Here's how the part is built. I have some questions about the finished solid (model axes, mm). Give positions to 0.01 mm unless a question says otherwise; leave off trailing zeros. Loops run counter-clockwise (first coordinate to the right, second up) from the corner with the lowest first, then second, coordinate; pieces in that order, holes last. Notation, with made-up numbers: (-24.75, 25) - (34.25, 25) arc R22 cw to (34.25, 40) - close; hole circle Ø8 at (77.5, 5.25). An arc over 180 degrees is marked (long way). Put each result on its own line as item: value. Start each with the question number.
from build123d import *

# Parameters (mm, degrees)
CROQUIS1_W              = 33.201006025
CROQUIS1_H              = 22.978323476
SALIENTE_EXTRUIR1_DEPTH = 2
CROQUIS3_R              = 1.35
CROQUIS3_R_2            = 1.347868192
CROQUIS3_R_3            = 1.352554563
CORTAR_EXTRUIR2_DEPTH   = 41.51793761
REDONDEO2_R             = 4
REDONDEO3_R             = 4
CORTAR_EXTRUIR3_DEPTH   = 41.51793761


with BuildPart() as part:
    # Croquis1 → Saliente-Extruir1 (new body)
    with BuildSketch(Plane.XY):
        with Locations((16.58985656, 11.664742893)):
            Rectangle(CROQUIS1_W, CROQUIS1_H)
    extrude(amount=SALIENTE_EXTRUIR1_DEPTH)

    # Croquis3 → Cortar-Extruir2 (cut, through all)
    with BuildSketch(Plane(origin=(0, 0, 0), x_dir=(-1, 0, 0), z_dir=(0, 0, -1))):
        with Locations((-30.114791782, 19.441420757)):
            Circle(CROQUIS3_R)
        with Locations((-3.064921335, 19.441420756)):
            Circle(CROQUIS3_R_2)
        with Locations((-3.064921337, 3.888065031)):
            Circle(CROQUIS3_R_3)
        with Locations((-30.114791782, 3.888065031)):
            Circle(CROQUIS3_R)
    extrude(amount=-CORTAR_EXTRUIR2_DEPTH, mode=Mode.SUBTRACT)

    # Redondeo2
    redondeo2_edges = [part.edges().sort_by_distance(p)[0] for p in [
        (33.190359572, 23.153904631, 1),
        (33.190359572, 0.175581155, 1),
    ]]
    fillet(redondeo2_edges, radius=REDONDEO2_R)

    # Redondeo3
    redondeo3_edges = [part.edges().sort_by_distance(p)[0] for p in [
        (-0.010646453, 23.153904631, 1),
        (-0.010646453, 0.175581155, 1),
    ]]
    fillet(redondeo3_edges, radius=REDONDEO3_R)

    # Croquis4 → Cortar-Extruir3 (cut, through all)
    with BuildSketch(Plane.XY.offset(2)):
        with BuildLine():
            Line((8.589856559, 18.464742893), (8.589856559, 19.664742893))
            Line((8.589856559, 19.664742893), (9.789856559, 19.664742893))
            ThreePointArc((9.789856559, 19.664742893), (7.741328422, 20.513271031), (8.589856559, 18.464742893))
        make_face()
        with BuildLine():
            Line((9.789856559, 19.664742893), (8.589856559, 19.664742893))
            Line((8.589856559, 19.664742893), (8.589856559, 18.464742893))
            ThreePointArc((8.589856559, 18.464742893), (9.438384697, 18.816214756), (9.789856559, 19.664742893))
        make_face()
        with BuildLine():
            ThreePointArc((9.789856559, 11.664742893), (9.438384697, 12.513271031), (8.589856559, 12.864742893))
            Line((8.589856559, 12.864742893), (8.589856559, 10.464742893))
            ThreePointArc((8.589856559, 10.464742893), (9.438384697, 10.816214756), (9.789856559, 11.664742893))
        make_face()
        with BuildLine():
            Line((8.589856559, 10.464742893), (8.589856559, 12.864742893))
            ThreePointArc((8.589856559, 12.864742893), (7.389856559, 11.664742893), (8.589856559, 10.464742893))
        make_face()
        with BuildLine():
            ThreePointArc((9.789856559, 3.664742893), (9.438384697, 4.513271031), (8.589856559, 4.864742893))
            Line((8.589856559, 4.864742893), (8.589856559, 3.664742893))
            Line((8.589856559, 3.664742893), (9.789856559, 3.664742893))
        make_face()
        with BuildLine():
            Line((8.589856559, 3.664742893), (8.589856559, 4.864742893))
            ThreePointArc((8.589856559, 4.864742893), (7.741328422, 2.816214756), (9.789856559, 3.664742893))
            Line((9.789856559, 3.664742893), (8.589856559, 3.664742893))
        make_face()
        with BuildLine():
            ThreePointArc((17.789856559, 3.664742893), (16.589856559, 4.864742893), (15.389856559, 3.664742893))
            Line((15.389856559, 3.664742893), (17.789856559, 3.664742893))
        make_face()
        with BuildLine():
            Line((17.789856559, 3.664742893), (15.389856559, 3.664742893))
            ThreePointArc((15.389856559, 3.664742893), (16.589856559, 2.464742893), (17.789856559, 3.664742893))
        make_face()
        with BuildLine():
            ThreePointArc((25.789856559, 3.664742893), (25.438384697, 4.513271031), (24.589856559, 4.864742893))
            Line((24.589856559, 4.864742893), (24.589856559, 3.664742893))
            Line((24.589856559, 3.664742893), (23.389856559, 3.664742893))
            ThreePointArc((23.389856559, 3.664742893), (24.589856559, 2.464742893), (25.789856559, 3.664742893))
        make_face()
        with BuildLine():
            Line((24.589856559, 3.664742893), (24.589856559, 4.864742893))
            ThreePointArc((24.589856559, 4.864742893), (23.741328422, 4.513271031), (23.389856559, 3.664742893))
            Line((23.389856559, 3.664742893), (24.589856559, 3.664742893))
        make_face()
        with BuildLine():
            ThreePointArc((25.789856559, 11.664742893), (25.438384697, 12.513271031), (24.589856559, 12.864742893))
            Line((24.589856559, 12.864742893), (24.589856559, 10.464742893))
            ThreePointArc((24.589856559, 10.464742893), (25.438384697, 10.816214756), (25.789856559, 11.664742893))
        make_face()
        with BuildLine():
            Line((24.589856559, 10.464742893), (24.589856559, 12.864742893))
            ThreePointArc((24.589856559, 12.864742893), (23.389856559, 11.664742893), (24.589856559, 10.464742893))
        make_face()
        with BuildLine():
            ThreePointArc((25.789856559, 19.664742893), (24.589856559, 20.864742893), (23.389856559, 19.664742893))
            Line((23.389856559, 19.664742893), (24.589856559, 19.664742893))
            Line((24.589856559, 19.664742893), (24.589856559, 18.464742893))
            ThreePointArc((24.589856559, 18.464742893), (25.438384697, 18.816214756), (25.789856559, 19.664742893))
        make_face()
        with BuildLine():
            Line((24.589856559, 19.664742893), (23.389856559, 19.664742893))
            ThreePointArc((23.389856559, 19.664742893), (23.741328422, 18.816214756), (24.589856559, 18.464742893))
            Line((24.589856559, 18.464742893), (24.589856559, 19.664742893))
        make_face()
        with BuildLine():
            ThreePointArc((17.789856559, 19.664742893), (16.589856559, 20.864742893), (15.389856559, 19.664742893))
            Line((15.389856559, 19.664742893), (17.789856559, 19.664742893))
        make_face()
        with BuildLine():
            Line((17.789856559, 19.664742893), (15.389856559, 19.664742893))
            ThreePointArc((15.389856559, 19.664742893), (16.589856559, 18.464742893), (17.789856559, 19.664742893))
        make_face()
    extrude(amount=-CORTAR_EXTRUIR3_DEPTH, mode=Mode.SUBTRACT)


solid = part.part
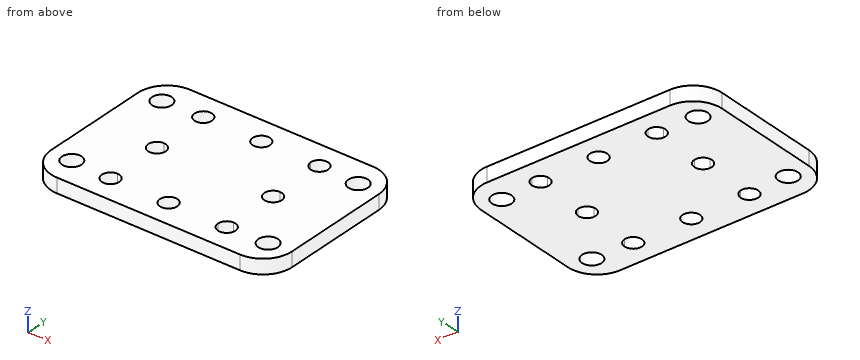
1) Suppose I cut it at A-A on x = 16. Please give me the cut outline in (y, z).
2) Suppose I cut it at D-D on y = 21.5. Please give me the cut outline in (x, z), plus the area to 3 significant figures.
3) Suppose I cut it at B-B on z = 1.3. Give the number of separate pieces and of enclosed holes in the cut face, plus the area to 3 significant figures.
4) I need wall thicknesses on line 1 (Y direction, x = 7.5, z = 0.1); line 2 (Y direction, x = 31, z = 0.4); line 3 (X direction, y = 20.25, z = 0.35). Which ranges of each line are inside material? Lowest first, please.
5) Suppose I cut it at C-C on x = 8. Please give me the cut outline in (y, z).
Ans:
1. outline: (0.18, 0) - (2.62, 0) - (2.62, 2) - (0.18, 2) - close; (4.71, 0) - (18.62, 0) - (18.62, 2) - (4.71, 2) - close; (20.71, 0) - (23.15, 0) - (23.15, 2) - (20.71, 2) - close
2. outline: (0.75, 0) - (32.43, 0) - (32.43, 2) - (0.75, 2) - close
2. area: 63.4 mm²
3. separate pieces: 1
3. enclosed holes: 12
3. area: 690 mm²
4. line 1: y = 0.18 to 3.16, 4.17 to 11.16, 12.17 to 19.16, 20.17 to 23.15
4. line 2: y = 0.61 to 2.87, 4.91 to 18.42, 20.46 to 22.72
4. line 3: x = 0.14 to 1.99, 4.14 to 7.54, 9.64 to 15.54, 17.64 to 23.54, 25.64 to 29.03, 31.2 to 33.04
5. outline: (0.18, 0) - (2.62, 0) - (2.62, 2) - (0.18, 2) - close; (4.71, 0) - (10.62, 0) - (10.62, 2) - (4.71, 2) - close; (12.71, 0) - (18.62, 0) - (18.62, 2) - (12.71, 2) - close; (20.71, 0) - (23.15, 0) - (23.15, 2) - (20.71, 2) - close
